Geometry: final body of the model. Coordinates: model frame, mm. A direction names the side the tool comes from. Give positions to 0.01 mm unless a question says otherwise; leave off trailing zeros. Write each loop counter-clockwise with the first axis right and the second up, starting at its lowest first coordinate (ties: lowest second). Pieces come first, ordered by that corner, then holes. Notation, with made-up numbers: M -2,48.5 L 49,48.5 A13 cw 49,67.5 Z; hole C 15.25,42.5 d4. An arc over 180 degrees is marked long. Answer as a JSON object with one key per item and string values.
from build123d import *

# Parameters (mm, degrees)
SKETCH2_R           = 22.15
SKETCH2_R_2         = 9.45
BOSS_EXTRUDE2_DEPTH = 15
SKETCH3_R           = 22.15
BOSS_EXTRUDE3_DEPTH = 2
CUT_EXTRUDE1_DEPTH  = 15
CIRPATTERN1_COUNT   = 3
CUT_EXTRUDE2_DEPTH  = 17
CIRPATTERN2_COUNT   = 3


with BuildPart() as part:
    # Sketch2 → Boss-Extrude2 (new body)
    with BuildSketch(Plane(origin=(0, 0, 0), x_dir=(1, 0, 0), z_dir=(0, 1, 0))):
        Circle(SKETCH2_R)
        Circle(SKETCH2_R_2, mode=Mode.SUBTRACT)
    extrude(amount=BOSS_EXTRUDE2_DEPTH)

    # Sketch3 → Boss-Extrude3 (add)
    with BuildSketch(Plane.XZ):
        Circle(SKETCH3_R)
    extrude(amount=BOSS_EXTRUDE3_DEPTH)

    # Sketch4 → Cut-Extrude1 (cut)
    with BuildSketch(Plane(origin=(0, 15, 0), x_dir=(1, 0, 0), z_dir=(0, 1, 0))):
        with BuildLine():
            Line((-1.6875, 22.085625274), (-1.6875, 9.298109687))
            ThreePointArc((-1.6875, 9.298109687), (0, 9.45), (1.6875, 9.298109687))
            Line((1.6875, 9.298109687), (1.6875, 22.085625274))
            ThreePointArc((1.6875, 22.085625274), (0, 22.15), (-1.6875, 22.085625274))
        make_face()
    cut_extrude1 = extrude(amount=-CUT_EXTRUDE1_DEPTH, mode=Mode.SUBTRACT)

    # CirPattern1: Cut-Extrude1 ×3 about axis
    cirpattern1_axis = Axis((0, 0, 0), (0, 1, 0))
    for i in range(1, CIRPATTERN1_COUNT):
        add(cut_extrude1.rotate(cirpattern1_axis, i * 360 / CIRPATTERN1_COUNT), mode=Mode.SUBTRACT)

    # Sketch6 → Cut-Extrude2 (cut)
    with BuildSketch(Plane(origin=(0, 15, 0), x_dir=(1, 0, 0), z_dir=(0, 1, 0))):
        with BuildLine():
            Line((-20.384492706, -8.665734654), (-10.089313607, -2.72181023))
            ThreePointArc((-10.089313607, -2.72181023), (-9.04996547, 5.225), (-2.6875, 10.098507006))
            Line((-2.6875, 10.098507006), (-2.6875, 21.986355854))
            ThreePointArc((-2.6875, 21.986355854), (-19.182462694, 11.075), (-20.384492706, -8.665734654))
        make_face()
    cut_extrude2 = extrude(amount=-CUT_EXTRUDE2_DEPTH, mode=Mode.SUBTRACT)

    # CirPattern2: Cut-Extrude2 ×3 about axis
    cirpattern2_axis = Axis((0, 0, 0), (0, 1, 0))
    for i in range(1, CIRPATTERN2_COUNT):
        add(cut_extrude2.rotate(cirpattern2_axis, i * 360 / CIRPATTERN2_COUNT), mode=Mode.SUBTRACT)


solid = part.part
1) Set-up query: faces 5 (the flat face through (-12.48, 6.62, 10.31)), 6 (the flat face through (0, 0, 0)), 7 (the flat face through (1.688, 8, -16)), 8 (the flat face through (2.688, 7, -16)), 9 (the flat face through (0, 15, 10)). Return all of +Z, -Z, +X, -X, +Y, -Y with unobstructed straight access to the full face (end or side cutting, diameter ignored); none if empty.
Geometry check:
{"face 5": "+Z, +Y, -Y", "face 6": "+Y", "face 7": "-Z, +Y", "face 8": "-Z, +X, +Y, -Y", "face 9": "+Z, -Z, +X, -X, +Y"}
2) Cut plane B-B on z = -17.5. Return loops of the section in (x, y), and give its area (4 significant figures).
Geometry check:
{"outline": "M -2.69,-2 L 2.69,-2 L 2.69,15 L 1.69,15 L 1.69,0 L -1.69,0 L -1.69,15 L -2.69,15 Z", "area": "40.75 mm2"}
3) Cut plane C-C on x = -4. Return loops of the section in (y, z), and give its area (3 significant figures).
Geometry check:
{"outline": "M -2,-9.65 L 15,-9.65 L 15,-8.56 L 0,-8.56 L 0,8.56 L 15,8.56 L 15,9.65 L -2,9.65 Z", "area": "71.4 mm2"}
4) Pull-direction query (Z, two-part tool) for faces 1 (the flat face through (-9, 15, -4)), 2 (the cylindrical face through (8.24, 7.4, -4.63)), 3 (the cylindrical face through (-8.13, 7.4, -4.82)), 4 (the flat face through (12.62, 6.62, 10.39)); classes: pulls with the +Z half, pulls with the -Z half, needs draft (parallel to the pull), parting line crosses it, or undercut.
Geometry check:
{"face 1": "needs draft", "face 2": "undercut", "face 3": "undercut", "face 4": "pulls with the +Z half"}
5) Contact query for flat-ended pins moving along their axis: P1, Ø10, axis at y = 0, z = 1.5, coming from the -X side; P2, Ø4, axis at x = -3, y = 5, coming from the -Z side; P3, Ø4, axis at y = 10, z = 7.5, coming from the +X side. Output: stop coordinate, or through.
Geometry check:
{"P1": "stops at x = -16.63", "P2": "stops at z = -22.09", "P3": "stops at x = 20.38"}
6) Line query: line 1 (X direction, y = 9.75, z = 7); line 2 (X direction, y = 2.25, z = 0); line 3 (Z direction, x = -2, y = 11). Output: solid intervals per line, ascending. Write a range as from..to.
Geometry check:
{"line 1": "x = -17.5..-15.5, -8.75..-6.35, 6.35..8.75, 15.5..17.5", "line 2": "x = -10.45..-9.45, 9.45..10.45", "line 3": "z = -22.06..-9.24, 9.24..10.26"}
7) Cut plane A-A on y = 8. Return loops of the section in (x, z).
Geometry check:
{"outline": "M -20.38,8.67 L -10.09,2.72 A10.45 ccw -2.69,-10.1 L -2.69,-21.99 A22.15 ccw -1.69,-22.09 L -1.69,-9.3 A9.45 cw -8.9,3.19 L -19.97,9.58 A22.15 ccw Z; M -18.28,12.5 L -7.21,6.11 A9.45 cw 7.21,6.11 L 18.28,12.5 A22.15 ccw 17.7,13.32 L 7.4,7.38 A10.45 ccw -7.4,7.38 L -17.7,13.32 A22.15 ccw Z; M 1.69,-22.09 A22.15 ccw 2.69,-21.99 L 2.69,-10.1 A10.45 ccw 10.09,2.72 L 20.38,8.67 A22.15 ccw 19.97,9.58 L 8.9,3.19 A9.45 cw 1.69,-9.3 Z"}
